Input: part model. Units: mm. Frame: model coordinates. Coordinates: 2 decimals unless noted, no trailing zeros. Write each loop counter-clockwise with the first axis right and the second up, starting at its lowest first coordinate (ties: lowest second). Pieces come first, ordered by that corner, then holes. Notation, with made-up numbers: (-38.5, -23.75) - (-11.5, -23.75) arc R25 cw to (-11.5, -6.75) - close; hole circle Ø1 at (83, 15). An arc over 180 degrees is marked (long way). Use a Markdown table: item, result. Add a question column.
Q1. Section query B-B (z = -277). Return the cut outline in (x, y) (3 decimals), then the cut area to 3 significant figures.
Q2. Material intervals for probe 1 along X at (y, z) = (5.5, -165.5) (3 decimals); probe 2 along Z at (x, y) = (-11.25, -1) (3 decimals), sorted ascending. Write a range as from..to.
Q3. Section query C-C (y = -5.25). Return the cut outline in (x, z) (3 decimals).
Q4. Section query A-A (x = -2.25). Return the cut outline in (y, z) (3 decimals).
Q5. Pin query (flat end, axial travel): P1, Ø1.5, axis at x = -0.5, y = 7.5, coming from the -Z side. Return the tip coordinate at first contact, or that it passes through.
from build123d import *

# Parameters (mm, degrees)
SKETCH1_W           = 25.4
SKETCH1_H           = 25.4
SKETCH1_W_2         = 19.05
SKETCH1_H_2         = 19.05
BOSS_EXTRUDE1_DEPTH = 323.85
SKETCH2_W           = 25.4
SKETCH2_H           = 29.329393675
CUT_EXTRUDE1_DEPTH  = 281.965076789


with BuildPart() as part:
    # Sketch1 → Boss-Extrude1 (new body)
    with BuildSketch(Plane.XY):
        Rectangle(SKETCH1_W, SKETCH1_H)
        Rectangle(SKETCH1_W_2, SKETCH1_H_2, mode=Mode.SUBTRACT)
    boss_extrude1 = extrude(amount=BOSS_EXTRUDE1_DEPTH)

    # Sketch2 → Cut-Extrude1 (cut, through all)
    with BuildSketch(Plane(origin=(0, 137.056163508, 237.388238686), x_dir=(1, 0, 0), z_dir=(0, 0.4999999999999889, 0.866025403784445))):
        with Locations((0, -158.25882579)):
            Rectangle(SKETCH2_W, SKETCH2_H)
    cut_extrude1 = extrude(amount=CUT_EXTRUDE1_DEPTH, mode=Mode.SUBTRACT)

    # Mirror2: Boss-Extrude1, Cut-Extrude1 across plane
    add(boss_extrude1.mirror(Plane.XY))
    add(cut_extrude1.mirror(Plane.XY), mode=Mode.SUBTRACT)


solid = part.part
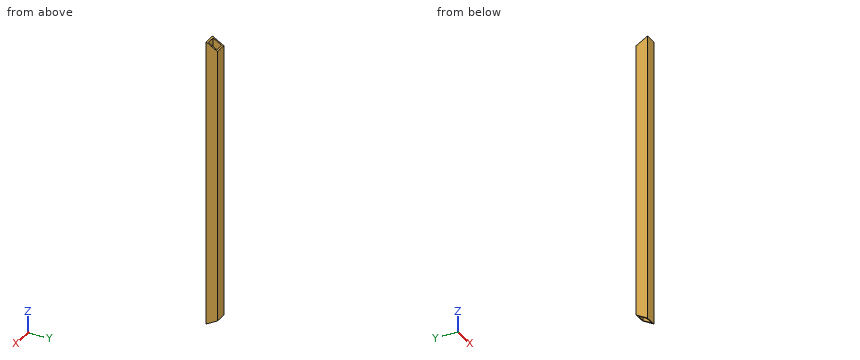
Values follow:
| question | item | result |
|---|---|---|
| 1 | outline | (-12.7, -12.7) - (12.7, -12.7) - (12.7, 12.7) - (-12.7, 12.7) - close; hole (-9.525, -9.525) - (9.525, -9.525) - (9.525, 9.525) - (-9.525, 9.525) - close |
| 1 | area | 282 mm2 |
| 2 | probe 1 | -12.7..-9.525, 9.525..12.7 |
| 2 | probe 2 | -317.095..317.095 |
| 3 | outline | (-12.7, -319.549) - (-9.525, -319.549) - (-9.525, 319.549) - (-12.7, 319.549) - close; (9.525, -319.549) - (12.7, -319.549) - (12.7, 319.549) - (9.525, 319.549) - close |
| 4 | outline | (-12.7, -323.85) - (-9.525, -322.017) - (-9.525, 322.017) - (-12.7, 323.85) - close; (9.525, -311.018) - (12.7, -309.185) - (12.7, 309.185) - (9.525, 311.018) - close |
| 5 | P1 | through |
